Verification items for the finished model (mm, model axes). A direction names the side the tool comes from. Round coordinates to 2 decimals unless told otherwise and drop trailing zeros. Order: outer loops, then holes, each group sorted by start corner. A loop starts at its lowest first (then second) coordinate and runs counter-clockwise, first axis right, second up. Notation, with made-up numbers: M 31.5,64 L 49.5,64 A12 ccw 49.5,73 Z; hole C -1.75,0.5 d8. An arc over 180 degrees is marked long. Use one line per item in the form item = value. Start each with the question number.
Item 1: Cross-section at A-A on z = 36. Enter the section's corners in (x, y).
Item 2: Go/stop test with a flat-tipped pin: pin 1 Ø4 at (x, y) = (-28, -7.5) entering from -Z. Record where the tip stops, or that it passes through.
Item 3: Thickness scan on probe 1 along X at (y, z) = (-35, 29); probe 2 along Z at (x, y) = (-22, -22). Record the ranges inside material, lowest first. Write a range as [from, to].
Item 4: Cross-section at B-B on y = -5. Enter the section's corners in (x, z).
Item 5: Tool access check on faces 4 (the flat face through (-4, -48, 40)), 5 (the flat face through (-1, 47.5, 21)). Record the directions out of +Z, -Z, +X, -X, +Y, -Y that give a thin tool (end or side, any length) a straight path to the whole face; none if there is none.
Item 6: Release check for a two-part mould opening along X. For faces 1 (the flat face through (-1, -50, 20)), 2 (the flat face through (47.5, -1, 21)), 3 (the flat face through (50, -1, 20)) record: +X half, -X half, draft (parallel to the pull), parting line (faces both ways), or undercut.
from build123d import *

# Parameters (mm, degrees)
F0_W     = 100
F0_H     = 100
F1_DEPTH = 25
F2_T     = -2.5
F3_DEPTH = 40
F4_T     = -2.5


with BuildPart() as f1:
    # F0 (on Top) → F1 (new body)
    with BuildSketch(Plane.XY):
        Rectangle(F0_W, F0_H)
    extrude(amount=F1_DEPTH)

    # F2
    f2_openings = [f1.faces().sort_by_distance(p)[0] for p in [
        (0, 0, 25),
    ]]
    offset(amount=F2_T, openings=f2_openings)

    # F0 (on Top) → F3 (join)
    with BuildSketch(Plane.XY):
        Rectangle(F0_W, F0_H)
    extrude(amount=F3_DEPTH)

    # F4
    f4_openings = [f1.faces().sort_by_distance(p)[0] for p in [
        (0, 0, 40),
    ]]
    offset(amount=F4_T, openings=f4_openings)


solid = f1.part
Output values:
q1.outline = M -50,-50 L 50,-50 L 50,50 L -50,50 Z; hole M -47.5,-47.5 L 47.5,-47.5 L 47.5,47.5 L -47.5,47.5 Z
q2.pin_1 = 0
q3.probe_1 = [-50, -47.5], [47.5, 50]
q3.probe_2 = [0, 2.5]
q4.outline = M -50,0 L 50,0 L 50,40 L 47.5,40 L 47.5,2.5 L -47.5,2.5 L -47.5,40 L -50,40 Z
q5.face_4 = +Z, +X, -X, +Y, -Y
q5.face_5 = +Z
q6.face_1 = draft
q6.face_2 = undercut
q6.face_3 = +X half
